Check sheet for the modelled part. Datum: model origin and axes. Units: mm. Face numbers are marked on the shaded views. Round coordinates to 2 decimals unless told otherwise and drop trailing zeros. Loops run counter-clockwise (first coordinate to the right, second up) from the corner with the lowest first, then second, coordinate; pieces in that order, holes last. Notation, with made-up numbers: (-37, 1) - (20, 1) arc R27 ccw to (20, 18) - close; hole circle Ø1 at (-4, -38.5). An arc over 180 degrees is marked (long way). Put each result on its own line as item: value. Start each with the question number.
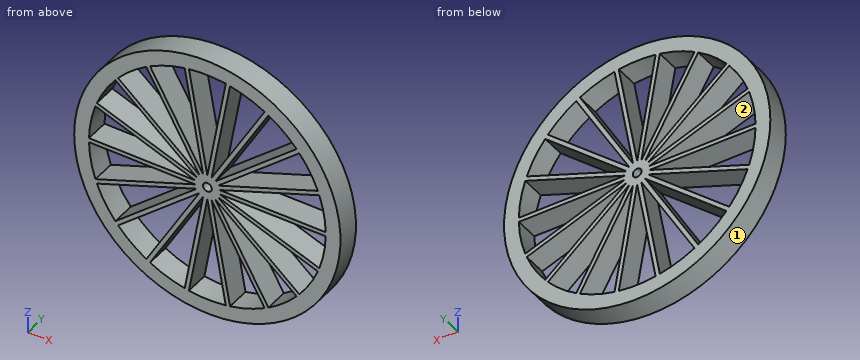
Autodesk Inventor part; units mm, degrees
ref_plane "YZ Plane" through (0, 0, 0) normal (1, 0, 0) x (0, 1, 0)
ref_plane "XZ Plane" through (0, 0, 0) normal (0, 1, 0) x (-1, 0, 0)
ref_plane "XY Plane" through (0, 0, 0) normal (0, 0, 1) x (1, 0, 0)
sketch "Sketch1" plane through (0, 0, 0) normal (0, 1, 0) x (-1, 0, 0)
  circle A0 centre (0, 0) radius 45
  circle A1 centre (0, 0) radius 40
  line L0 (40, 0) -> (-70, 0)
  line L1 (-39.9934, 0.7273) -> (39.9934, 0.7273)
  point P0 (-40, 0)
  dimension "d0" = 90
  dimension "d1" = 80
extrude "Extrusion1" add sketch "Sketch1" along normal blind 8
extrude "Extrusion2" add sketch "Sketch1" along normal blind 8 contours A1 L1 L0
pattern_circular "Circular Pattern1" count 18 over 360 about axis through (0, -10, 0) along (0, 1, 0) of "Extrusion2"
sketch "Sketch2" plane through (0, 8, 0) normal (0, 1, 0) x (1, 0, 0)
  circle A0 centre (0, 0) radius 1.5
  dimension "d9" = 3
hole "Hole1" at (0, 8, 0) direction (0, -1, 0) diameter 3 end through all
thread "Thread1"
properties part number "Tyres"
Q1. Cross-section at C-C on z = -37. Enter the section's corners in (x, y).
Q2. Cross-section at A-A on z = -20.5. State how many separate pieces and enclosed holes the cut face has, and give its area (3 significant figures).
Q3. Draft check along X on the marked faces 1 and 2. Enter one of: +X half, -X half, draft (parallel to the pull), parting line (faces both ways), or undercut.
Q4. Depth check by flat-ended pin: pin 1 Ø4 at (x, y) = (27.5, 3) entering from -Z; pin 2 Ø4 at (x, y) = (4, 5.5) entering from -Z; pin 3 Ø4 at (x, z) = (6.5, -29.5) entering from +Y; pin 4 Ø2 at (y, z) = (7, -11.5) entering from -X. Enter the tip coordinate at first touch or a pass-through.
Q5. Material ranges on line 1 (X direction, y = 2, z = -34); line 2 (X direction, y = 3, z = 30); line 3 (X direction, y = 4.5, z = 0), recorded low to high. Write a range as from..to.
Q6. Cross-section at B-B on x = 28. Enter the section's corners in (y, z), and give its area (3 significant figures).
Answer list:
1. outline: (-25.61, 0) - (-15.2, 0) - (-15.2, 8) - (-25.61, 8) - close; (-7.26, 0) - (-5.79, 0) - (-5.79, 8) - (-7.26, 8) - close; (5.79, 0) - (7.26, 0) - (7.26, 8) - (5.79, 8) - close; (15.2, 0) - (25.61, 0) - (25.61, 8) - (15.2, 8) - close
2. separate pieces: 8
2. enclosed holes: 0
2. area: 178 mm2
3. face 1: parting line
3. face 2: undercut
4. pin 1: stops at z = -37.08
4. pin 2: stops at z = -44.96
4. pin 3: stops at y = 8
4. pin 4: stops at x = -43.76
5. line 1: x = -29.48..-21.07, -20.47..-18.79, -6.73..-5.26, 5.26..6.73, 18.79..20.47, 21.07..29.48
5. line 2: x = -33.54..-26.46, -18.16..-16.48, -6.03..-4.55, 4.55..6.03, 16.48..18.16, 26.46..33.54
5. line 3: x = -45..-1.5, 1.5..45
6. outline: (0, -35.23) - (8, -35.23) - (8, -28.57) - (0, -28.57) - close; (0, -24.44) - (8, -24.44) - (8, -22.55) - (0, -22.55) - close; (0, -10.97) - (8, -10.97) - (8, -9.42) - (0, -9.42) - close; (0, -0.73) - (8, -0.73) - (8, 0.73) - (0, 0.73) - close; (0, 9.42) - (8, 9.42) - (8, 10.97) - (0, 10.97) - close; (0, 22.55) - (8, 22.55) - (8, 24.44) - (0, 24.44) - close; (0, 28.57) - (8, 28.57) - (8, 35.23) - (0, 35.23) - close
6. area: 173 mm2
